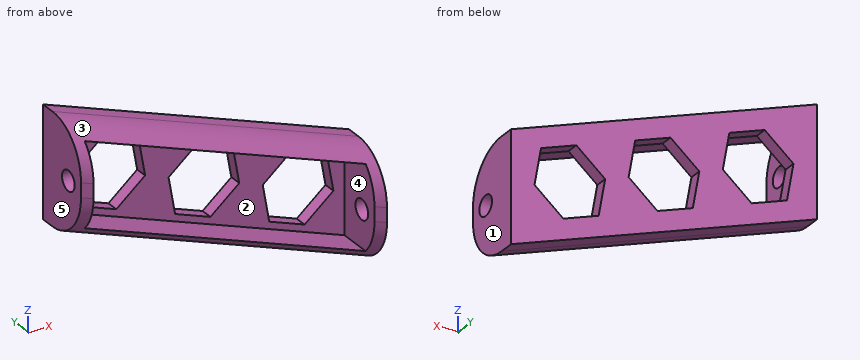
from build123d import *

# Parameters (mm, degrees)
F1_DEPTH    = 12
F2_T        = -2.5
F4_D        = 4
F4_DEPTH    = 6
F4_TIP      = 1.2017212381
F6_D        = 4
F6_DEPTH    = 6
F6_TIP      = 1.2017212381
F7_T1_DEPTH = 110
F7_T3_DEPTH = 110
F9_DEPTH    = 25


# Not quite as in the source:
# - a fillet or chamfer that OpenCascade refuses, or shapes differently, is made with other operations: its cross-section is extruded or revolved along the edge and cut away or added


with BuildPart() as f1:
    # F0 (on Front) → F1 (new body)
    with BuildSketch(Plane.XZ):
        Polygon((39.4877206884, 0), (-21.5922996627, 22.2313093162), (-21.5922996627, 0.2313093162), (39.4877206884, -22), align=None)
    extrude(amount=F1_DEPTH)

    # F2
    f2_openings = [f1.faces().sort_by_distance(p)[0] for p in [
        (8.947711, -12, 0.115655),
    ]]
    offset(amount=F2_T, openings=f2_openings)

    # F4
    with Locations(Plane(origin=(-21.5922996627, 0, 0), x_dir=(0, -1, 0), z_dir=(-1, 0, 0))):
        with Locations((8, 11.2313093162)):
            Hole(F4_D / 2, depth=F4_DEPTH)
            with Locations((0, 0, -(F4_DEPTH + F4_TIP / 2))):  # 118° drill point
                Cone(0, F4_D / 2, F4_TIP, mode=Mode.SUBTRACT)

    # F6
    with Locations(Plane.YZ.offset(39.4877206884)):
        with Locations((-8, -11)):
            Hole(F6_D / 2, depth=F6_DEPTH)
            with Locations((0, 0, -(F6_DEPTH + F6_TIP / 2))):  # 118° drill point
                Cone(0, F6_D / 2, F6_TIP, mode=Mode.SUBTRACT)

    # F7: fillet of radius 9 on 2 edges, made by hand

    # F7_s2 → F7_t1 (cut)
    with BuildSketch(Plane(origin=(56.0116188142, 0, -20.3865620214), x_dir=(0, 1, 0), z_dir=(-0.9396926208, 0, 0.3420201433))):
        with BuildLine():
            ThreePointArc((-3, -13.5055958894), (-9.3639610307, -10.8695569201), (-12, -4.5055958894))
            Line((-12, -4.5055958894), (-12, -13.5055958894))
            Line((-12, -13.5055958894), (-3, -13.5055958894))
        make_face()
    extrude(amount=F7_T1_DEPTH, mode=Mode.SUBTRACT)

    # F7_s4 → F7_t3 (cut)
    with BuildSketch(Plane(origin=(-40.2839057657, 0, 14.6621426187), x_dir=(0, 1, 0), z_dir=(0.9396926208, 0, -0.3420201433))):
        with BuildLine():
            ThreePointArc((-12, 1.8323582321), (-9.3639610307, -4.5316027985), (-3, -7.1676417679))
            Line((-3, -7.1676417679), (-12, -7.1676417679))
            Line((-12, -7.1676417679), (-12, 1.8323582321))
        make_face()
    extrude(amount=F7_T3_DEPTH, mode=Mode.SUBTRACT)

    # F8 (on face) → F9 (cut)
    with BuildSketch(Plane.XZ.offset(2.5)):
        Polygon((-8.5428162153, -0.4354697523), (-2.7932286645, 4.389007041), (-4.0965543521, 11.7805343179), (-11.1494675905, 14.3475848015), (-16.8990551413, 9.5231080082), (-15.5957294537, 2.1315807313), align=None)
        Polygon((10.2510362004, -7.2758726188), (16.0006237512, -2.4513958255), (14.6972980636, 4.9401314514), (7.6443848253, 7.507181935), (1.8947972745, 2.6827051417), (3.198122962, -4.7088221352), align=None)
        Polygon((29.0448886161, -14.1162754854), (34.7944761669, -9.2917986921), (33.4911504793, -1.9002714151), (26.438237241, 0.6667790685), (20.6886496902, -4.1576977248), (21.9919753777, -11.5492250017), align=None)
    extrude(amount=-F9_DEPTH, mode=Mode.SUBTRACT)


solid = f1.part
CAD build for the part. Positions are in the model's coordinates, mm. Face numbers are marked on the shaded views. A direction names the side the tool comes from. Round coordinates to 2 decimals unless told otherwise and drop trailing zeros. Order: outer loops, then holes, each group sorted by start corner. A loop starts at its lowest first (then second) coordinate and runs counter-clockwise, first axis right, second up. Notation, with made-up numbers: (53.25, 84.25) -> (105.25, 84.25) arc R28 ccw to (105.25, 122.25) -> close; hole circle Ø3 at (-17, 44.25). An arc over 180 degrees is marked (long way). Write each question's results on one line, items separated by ' | '.
1. Flat gauge pins, fed straight in: P1, Ø4, axis at x = 7.5, z = -3, coming from the -Y side; P2, Ø1, axis at x = 28, z = -15.5, coming from the -Y side; P3, Ø2, axis at x = 28, y = -1.5, coming from the +Z side. Where does each tip first touch, or does it go through?
Findings below:
P1: passes through | P2: stops at y = -9.22 | P3: stops at z = 4.55
2. Cut at B-B (y = -5.25). Give the cut face in (x, z).
Findings below:
outline: (-21.59, 0.54) -> (39.49, -21.7) -> (39.49, -0.3) -> (-21.59, 21.93) -> close; hole (-19.09, 1.98) -> (36.99, -18.43) -> (36.99, -1.75) -> (-19.09, 18.66) -> close
3. Pull direction Z, two halves, no side cores. Call the marked faces 3, 4 and 5: pulls with the +Z half, pulls with the -Z half, needs draft (parallel to the pull), parting line crosses it, or undercut.
Findings below:
face 3: pulls with the +Z half | face 4: undercut | face 5: needs draft
4. Cut at A-A (y = -8.25). Give the cut face in (x, z), plus the area to 3 significant figures.
Findings below:
outline: (-21.59, 2.03) -> (39.49, -20.2) -> (39.49, -12.98) -> (36.99, -12.98) -> (36.99, -18.43) -> (-19.09, 1.98) -> (-19.09, 9.25) -> (-21.59, 9.25) -> close; (-21.59, 13.22) -> (-19.09, 13.22) -> (-19.09, 18.66) -> (36.99, -1.75) -> (36.99, -9.02) -> (39.49, -9.02) -> (39.49, -1.8) -> (-21.59, 20.43) -> close | area: 169 mm²
5. Wall check: line 1 along Y through (x, z) = (-10, 14.5); line 2 along X through (y, z) = (-9.5, 14); line 3 along Z through (x, y) = (-13.5, -3.5). Give the ranges that are in metal, low to high. Write a range as [from, to].
Findings below:
line 1: y = [-2.5, 0] | line 2: x = [-21.59, -19.09] | line 3: z = [-2.7, -0.05], [16.63, 19.27]
6. Cut at C-C (z = 3.5). Count the separate pieces of the cut face and the enclosed holes in it, plus the area to 3 significant figures.
Findings below:
separate pieces: 3 | enclosed holes: 0 | area: 122 mm²
7. 3-axis set-ups, long thin cutter, end or side, ignore diameter. For the marked faces 1 and 2: which of +Z, -Z, +X, -X, +Y, -Y reach the whole face in a straight line?
Findings below:
face 1: +Z, -Z, +X, +Y, -Y | face 2: -Y
